Autodesk Inventor part; units mm, degrees
ref_plane "Work Plane1" through (0, 0, 330) normal (0, 0, 1) x (1, 0, 0)
ref_plane "YZ Plane" through (0, 0, 0) normal (1, 0, 0) x (0, 1, 0)
ref_plane "XZ Plane" through (0, 0, 0) normal (0, 1, 0) x (-1, 0, 0)
sketch "Sketch1" plane through (0, 0, 0) normal (0, 0, 1) x (1, 0, 0)
  line L0 (-7.5, 2.9) -> (7.5, 2.9)
  line L1 (7.5, 2.9) -> (7.5, -2.9)
  line L2 (7.5, -2.9) -> (-7.5, -2.9)
  line L3 (-7.5, -2.9) -> (-7.5, 2.9)
  line L4 (-7.5, 2.9) -> (7.5, -2.9) construction
  line L5 (7.5, 2.9) -> (-7.5, -2.9) construction
  line L6 (-12.5, 7.5) -> (12.5, 7.5)
  line L7 (12.5, 7.5) -> (12.5, -7.5)
  line L8 (12.5, -7.5) -> (-12.5, -7.5)
  line L9 (-12.5, -7.5) -> (-12.5, 7.5)
  line L10 (-12.5, 7.5) -> (12.5, -7.5) construction
  line L11 (12.5, 7.5) -> (-12.5, -7.5) construction
  line L12 (-7.5, 7.5) -> (-7.5, -7.5)
  point P0 (0, 0)
  point P1 (-7.5, 2.9)
  dimension "d0" = 15
  dimension "d1" = 5.8
  dimension "d2" = 25
  dimension "d3" = 15
extrude "Extrusion1" add sketch "Sketch1" along normal blind 500 contours L12 L6 L7 L8 L2 L1 L0
ref_plane "Work Plane1" through (0, 0, 330) normal (0, 0, 1) x (1, 0, 0)
sketch "Sketch2" plane through (0, 0, 330) normal (0, 0, 1) x (1, 0, 0)
  line L0 (-5, 7.5) -> (30, 7.5)
  line L1 (30, 7.5) -> (30, -7.5)
  line L2 (30, -7.5) -> (-5, -7.5)
  line L3 (-5, -7.5) -> (-5, 7.5)
  line L4 (12.5, -7.5) -> (12.5, 7.5)
  line L5 (-5, 7.5) -> (30, -7.5) construction
  line L6 (30, 7.5) -> (-5, -7.5) construction
  line L7 (12.5, 0) -> (30, 0)
  line L8 (30, 0) -> (30, 7.5)
  line L9 (30, 7.5) -> (12.5, 7.5)
  line L10 (12.5, 7.5) -> (12.5, 0)
  line L11 (7.5, -2.9) -> (-7.5, -2.9)
  line L12 (-7.5, -2.9) -> (-7.5, -7.5)
  line L13 (-7.5, -7.5) -> (12.5, -7.5)
  line L14 (12.5, -7.5) -> (12.5, 7.5)
  line L15 (12.5, 7.5) -> (-7.5, 7.5)
  line L16 (-7.5, 7.5) -> (-7.5, 2.9)
  line L17 (-7.5, 2.9) -> (7.5, 2.9)
  line L18 (7.5, 2.9) -> (7.5, -2.9)
  point P0 (0, 0)
  point P1 (12.5, -6.5)
  point P2 (12.5, 6.5)
  point P3 (12.5, 7.5)
  point P4 (12.5, 6.5)
  point P5 (30, 0)
  dimension "d8" = 35
extrude "Extrusion2" add sketch "Sketch2" against normal blind 25 contours L0 L1 L7 L4
fillet "Fillet2" radius 6 3 edges at (12.5, 3.75, 305) (12.5, 0, 317.5) (12.5, 3.75, 330)
sketch "Sketch4" plane through (-7.5, 7.5, 0) normal (0, 1, 0) x (1, 0, 0)
  line L0 (20, 0) -> (0, 0)
  line L1 (0, 0) -> (0, -500)
  line L2 (20, -500) -> (0, -500)
  line L3 (20, -336) -> (20, -500)
  arc A0 (26, -330) -> (20, -336) centre (26, -336) ccw
  line L4 (37.5, -330) -> (26, -330)
  line L5 (37.5, -330) -> (37.5, -305)
  line L6 (26, -305) -> (37.5, -305)
  arc A1 (20, -299) -> (26, -305) centre (26, -299) ccw
  line L7 (20, 0) -> (20, -299)
  circle A2 centre (30.5, -317.5) radius 1.65
  line L8 (20, 0) -> (20, -500)
  line L9 (20, -250) -> (51.65, -250)
  circle A3 centre (30.5, -142.5) radius 1.65
  point P0 (7.5, 0)
  point P1 (20, -181)
  point P2 (20, -144)
  point P3 (37.5, -317.5)
  point P4 (37.5, -142.5)
  dimension "d16" = 3.3
  dimension "d17" = 7
extrude "Extrusion4" cut sketch "Sketch4" against normal through all contours A2 | A3
chamfer "Chamfer1" distance 5 angle 45 2 edges at (30, 3.75, 330) (30, 3.75, 305)
sketch "Sketch5" plane through (18.5, 0, 305) normal (0, -1, 0) x (1, 0, 0)
  line L0 (11.5, -170) -> (6.5, -175)
  line L1 (11.5, -170) -> (11.5, -155)
  line L2 (6.5, -150) -> (11.5, -155)
  line L3 (0, -150) -> (6.5, -150)
  line L4 (0, -175) -> (0, -150)
  line L5 (6.5, -175) -> (0, -175)
  circle A0 centre (4.5, -162.5) radius 1.65
  circle A1 centre (4.5, 12.5) radius 1.65
  line L6 (11.5, 5) -> (6.5, 0)
  line L7 (11.5, 20) -> (11.5, 5)
  line L8 (6.5, 25) -> (11.5, 20)
  line L9 (0, 25) -> (6.5, 25)
  line L10 (0, 0) -> (0, 25)
  line L11 (6.5, 0) -> (0, 0)
  circle A2 centre (4.5, 12.5) radius 2.9
  circle A3 centre (4.5, -162.5) radius 2.9
  point P0 (-18.5, -305)
  dimension "d23" = 5.8
extrude "Extrusion5" cut sketch "Sketch5" against normal blind 3 contours A2 | A3
ref_plane "Work Plane3" through (0, 0, 250) normal (0, 0, -1) x (-1, 0, 0)
pattern_linear "Rectangular Pattern1" count 2 spacing 160 along (0, 0, 1) of "Extrusion2", "Fillet2", "Extrusion4", "Chamfer1", "Extrusion5"
mirror "Mirror1" about plane through (0, 0, 250) normal (0, 0, -1) of "Extrusion2", "Fillet2", "Extrusion4", "Chamfer1", "Extrusion5", "Rectangular Pattern1"
ref_plane "Work Plane4" through (0, 0, 250) normal (0, 0, 1) x (1, 0, 0)
sketch "Sketch6" plane through (0, 0, 250) normal (0, 0, 1) x (1, 0, 0)
  line L0 (12.5, 7.5) -> (12.5, -6)
  line L1 (12.5, -6) -> (12.5, 7.5)
  line L2 (12.5, 7.5) -> (12.5, -6)
  line L3 (12.5, -6) -> (12.5, 7.5)
  line L4 (12.5, 7.5) -> (12.5, -6)
  line L5 (12.5, -6) -> (12.5, 7.5)
  line L6 (12.5, 7.5) -> (12.5, -6)
  line L7 (12.5, -7.5) -> (12.5, 7.5)
  line L8 (12.5, -7.5) -> (12.5, 7.5)
  line L9 (12.5, -6) -> (12.5, 7.5)
  line L10 (12.5, 7.5) -> (32.5, 7.5)
  line L11 (32.5, 7.5) -> (32.5, -7.5)
  line L12 (32.5, -7.5) -> (12.5, -7.5)
  line L13 (12.5, -7.5) -> (12.5, 7.5)
  point P0 (0, 0)
  dimension "d29" = 20
extrude "Extrusion6" add sketch "Sketch6" along normal mid plane 20
sketch "Sketch7" plane through (0, 0, 250) normal (0, 0, 1) x (1, 0, 0)
  line L0 (-44.2383, 45.2094) -> (125.162, 45.2094)
  line L1 (125.162, 45.2094) -> (125.162, -53.1939)
  line L2 (125.162, -53.1939) -> (-44.2383, -53.1939)
  line L3 (-44.2383, -53.1939) -> (-44.2383, 45.2094)
  point P0 (0, 0)
extrude "Extrusion7" cut sketch "Sketch7" along normal through all
sketch "Sketch8" plane through (0, 0, 250) normal (0, 0, 1) x (1, 0, 0)
  line L0 (7.5, -2.9) -> (7.5, 2.9)
  line L1 (-7.5, -2.9) -> (7.5, -2.9)
  line L2 (-7.5, -7.5) -> (-7.5, -2.9)
  line L3 (32.5, -7.5) -> (-7.5, -7.5)
  line L4 (32.5, 7.5) -> (32.5, -7.5)
  line L5 (-7.5, 7.5) -> (32.5, 7.5)
  line L6 (-7.5, 2.9) -> (-7.5, 7.5)
  line L7 (7.5, 2.9) -> (-7.5, 2.9)
  line L8 (13.5, 3.5) -> (28.5, 3.5)
  line L9 (28.5, 3.5) -> (28.5, -3.5)
  line L10 (28.5, -3.5) -> (13.5, -3.5)
  line L11 (13.5, -3.5) -> (13.5, 3.5)
  line L12 (28.3, 3.3) -> (13.7, 3.3)
  line L13 (13.7, 3.3) -> (13.7, -3.3)
  line L14 (13.7, -3.3) -> (28.3, -3.3)
  line L15 (28.3, -3.3) -> (28.3, 3.3)
  point P0 (0, 0)
  point P1 (28.5, 0)
  point P2 (32.5, 0)
  dimension "d34" = 15
  dimension "d35" = 4
  dimension "d36" = 7
  dimension "d37" = 0.2
extrude "Extrusion8" add sketch "Sketch8" along normal blind 5.8 contours L15 L14 L13 L12
properties part number "GUIA DE TAPA PRINCIPAL"
Work out the finished part from the listing and answer in its coordinate system (mm). A direction names the side the tool comes from. Give positions to 0.01 mm unless a question says otherwise; leave off trailing zeros. Write each loop counter-clockwise with the first axis right and the second up, starting at its lowest first coordinate (ties: lowest second). Pieces come first, ordered by that corner, then holes. Notation, with made-up numbers: (25.25, 86) -> (73.25, 86) arc R15 cw to (73.25, 113) -> close; hole circle Ø8 at (-33.75, 12). An arc over 180 degrees is marked (long way). Write item = value, one per line.
Q1. Consider line 1 along Z through (x, y) = (19, 7.25); line 2 along Z through (x, y) = (20.5, 3.25); line 3 along Z through (x, y) = (23, 4.25). Determine where each line is inside the solid, lowest interval first.
Computed values:
line_1 = 10 to 35, 170 to 195, 240 to 250
line_2 = 10 to 35, 170 to 195, 240 to 255.8
line_3 = 10 to 20.85, 24.15 to 35, 170 to 180.85, 184.15 to 195, 240 to 250
Q2. A tool of negligible diameter and unlimited length cuts with its end or side. For faces 5 (the flat face through (22, 3, 184)), 6 (the cylindrical face through (14.304, -1.711, 22.759)), 7 (the flat face through (30, 4, 182)), 8 (the flat face through (28.3, 0, 253)), 9 (the flat face through (22, 5, 195)), from which of +Z, -Z, +X, -X, +Y, -Y can it reach the whole face along a straight path? Write none if from no direction.
Computed values:
face_5 = -Y
face_6 = -Z, +X, -Y
face_7 = -Z, +X, +Y, -Y
face_8 = +Z, +X, +Y, -Y
face_9 = +X, +Y, -Y
Q3. Section A-A on x = 3.5 is taken. Determine the outline of the cut face in (y, z), and give its area (3 significant figures).
Computed values:
outline = (-7.5, 0) -> (-2.9, 0) -> (-2.9, 250) -> (-7.5, 250) -> close; (2.9, 0) -> (7.5, 0) -> (7.5, 250) -> (2.9, 250) -> close
area = 2,300 mm^2
Q4. Section B-B on z = 144.5 is taken. Determine the outline of the cut face in (x, y), and give its area (3 significant figures).
Computed values:
outline = (-7.5, -7.5) -> (12.5, -7.5) -> (12.5, 7.5) -> (-7.5, 7.5) -> (-7.5, 2.9) -> (7.5, 2.9) -> (7.5, -2.9) -> (-7.5, -2.9) -> close
area = 213 mm^2
Q5. For a pull along Y with two mould halves and no side action, classify faces 1 (the flat face through (27, 4, 172)), 2 (the flat face through (0, -2.9, 123)), 3 (the flat face through (4, 7.5, 127)), 4 (the flat face through (0, 2.9, 123)) as pulls with the +Y half, pulls with the -Y half, needs draft (parallel to the pull), parting line crosses it, or undercut.
Computed values:
face_1 = needs draft
face_2 = undercut
face_3 = pulls with the +Y half
face_4 = undercut
Q6. Flat-ended cylindrical pins translate along their axes: pin 1 Ø5.5 at (x, z) = (23, 22.5) entering from -Y; pin 2 Ø5 at (x, y) = (23, 2.5) entering from -Z; pin 3 Ø2 at (y, z) = (-1.5, 157.5) entering from -X. Find the tip coordinate at first contact, or state that the pin passes through.
Computed values:
pin_1 = 3
pin_2 = 10
pin_3 = 7.5
